For this review, take the finished solid that the model builds, in its own axes (mm). Face numbers are marked on the shaded views. A direction names the side the tool comes from. Round coordinates to 2 decimals unless told otherwise and drop trailing zeros. Order: outer loops, then holes, each group sorted by start corner. A loop starts at its lowest first (then second) coordinate and runs counter-clockwise, first axis right, second up.
from build123d import *

# Parameters (mm, degrees)
BOSS_EXTRUDE2_DEPTH     = 234
SKETCH3_R               = 44.45
CUT_EXTRUDE1_DEPTH      = 78
BOSS_EXTRUDE3_DEPTH     = 33
CUT_EXTRUDE3_REACH      = 336.868
CUT_EXTRUDE3_END_RADIUS = 28.575


with BuildPart() as part:
    # Sketch1 → Boss-Extrude2 (new body)
    with BuildSketch(Plane.XY):
        with BuildLine():
            Line((28.35361426, 84), (28.35361426, 40.991869112))
            Line((28.35361426, 40.991869112), (99.35361426, 0))
            Line((99.35361426, 0), (112.35361426, 0))
            Line((112.35361426, 0), (112.35361426, 55.425))
            ThreePointArc((112.35361426, 55.425), (83.77861426, 84), (112.35361426, 112.575))
            Line((112.35361426, 112.575), (112.35361426, 168))
            ThreePointArc((112.35361426, 168), (52.95664464, 143.39696962), (28.35361426, 84))
        make_face()
    extrude(amount=BOSS_EXTRUDE2_DEPTH)

    # Sketch3 → Cut-Extrude1 (cut)
    with BuildSketch(Plane.XY.offset(234)):
        with Locations((112.35361426, 84)):
            Circle(SKETCH3_R)
    extrude(amount=-CUT_EXTRUDE1_DEPTH, mode=Mode.SUBTRACT)

    # Sketch4 → Boss-Extrude3 (add)
    with BuildSketch(Plane.XY.offset(234)):
        with BuildLine():
            Line((46.922945338, 83.090294344), (97.407186315, 147.707176139))
            Line((97.407186315, 147.707176139), (79.823205858, 161.445287327))
            ThreePointArc((79.823205858, 161.445287327), (46.160710957, 135.715563927), (29.338964881, 96.828405531))
            Line((29.338964881, 96.828405531), (46.922945338, 83.090294344))
        make_face()
    extrude(amount=BOSS_EXTRUDE3_DEPTH)

    # Cut-Extrude3: up to this cylinder (the profile starts outside it)
    cut_extrude3_end = Plane(origin=(112.35361426, 84, 56.053764), z_dir=(0, 0, -1)) * Cylinder(CUT_EXTRUDE3_END_RADIUS, 731.886, mode=Mode.PRIVATE)
    # Sketch5 → Cut-Extrude3 (cut, up to the surface)
    with BuildSketch(Plane(origin=(0, 168, 0), x_dir=(1, 0, 0), z_dir=(0, 1, 0)), mode=Mode.PRIVATE) as cut_extrude3_sk1:
        Polygon((112.35361426, -38), (112.35361426, -74.107528994), (93.35361426, -72.445244387), (93.35361426, -39.662284607), align=None)
    cut_extrude3_tool1 = extrude(cut_extrude3_sk1.sketch, amount=-CUT_EXTRUDE3_REACH, mode=Mode.PRIVATE) - cut_extrude3_end
    add(cut_extrude3_tool1.solids().sort_by_distance((103.006434, 168, 56.053764))[0], mode=Mode.SUBTRACT)


solid = part.part
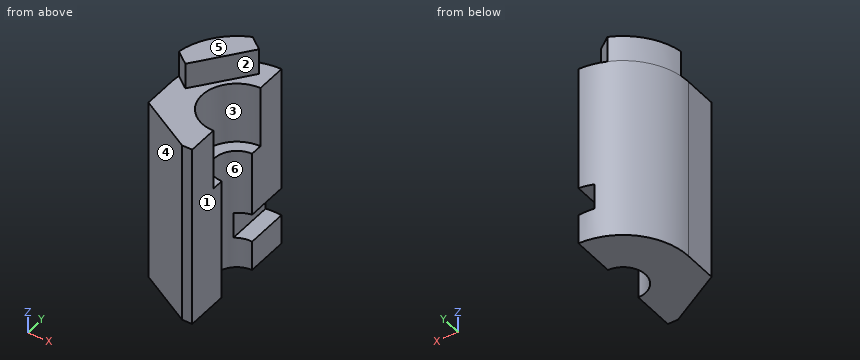
(1) Add section C-C on x = 40. Give the boundary of the cut face in (y, z).
(2) Draft analysis for pull direction Y (two halves, no side actions). For the marked faces 4, 5 and 6, state which applies: pulls with the +Y half, pulls with the -Y half, needs draft (parallel to the pull), parting line crosses it, or undercut.
(3) Add section A-A on z = 30.5. Give the boundary of the cut face in (x, y) (3 decimals), plus the area to 3 significant figures.
(4) Add section D-D on z = 63. Give the boundary of the cut face in (x, y) (3 decimals).
(5) Tool access review of the marked faces 1, 2 and 3: name each direction out of +Z, -Z, +X, -X, +Y, -Y from which nothing blocks a thin tool from reaching the whole face with its end or side.
(6) Wall thickness on L1, parallel to X at y = 82.5, z = 48.5; L2, parallel to Z at x = 40, y = 54; L3, parallel to Y at x = 76.5, z = 200: over which ranges is each line inside the solid? List them lowest first.
(7) Clearance check with flat-ended pins moving along their axes: P1, Ø10, axis at x = 45.5, z = 82.5, coming from the -Y side; P2, Ø2, axis at y = 146.5, z = 240, coming from the -X side; P3, Ø1.5, axis at x = 49, z = 154, coming from the +Y side. State where each tip first meets the part, or that it passes through.
(8) Add section B-B on y = 80. Give the boundary of the cut face in (x, z).
Here are the results:
1. outline: (34.27, 0) - (126.67, 0) - (126.67, 267) - (88.5, 267) - (88.5, 234) - (34.27, 234) - close
2. face 4: pulls with the -Y half
2. face 5: needs draft
2. face 6: undercut
3. outline: (28.354, 40.992) - (99.354, 0) - (112.354, 0) - (112.354, 55.425) arc R28.575 cw to (112.354, 112.575) - (112.354, 168) arc R84 ccw to (28.354, 84) - close
3. area: 9,860 mm2
4. outline: (28.354, 40.992) - (99.354, 0) - (112.354, 0) - (112.354, 55.425) arc R28.575 cw to (93.354, 105.343) - (93.354, 165.823) arc R84 ccw to (28.354, 84) - close
5. face 1: +Z, -Z, +X, +Y, -Y
5. face 2: +Z, +X, -Y
5. face 3: +Z, +X
6. L1: x = 28.35 to 83.82
6. L2: z = 0 to 234
6. L3: y = 13.19 to 57.73, 110.27 to 159.96
7. P1: stops at y = 28.21
7. P2: stops at x = 55.14
7. P3: stops at y = 140.01
8. outline: (28.35, 0) - (84.06, 0) - (84.06, 156) - (68.08, 156) - (68.08, 234) - (28.35, 234) - close
